```python
from build123d import *

# Parameters (mm, degrees)
SKETCH1_W           = 128.27
SKETCH1_H           = 143.764
BOSS_EXTRUDE1_DEPTH = 45.72
SKETCH3_W           = 115.57
SKETCH3_H           = 131.064
CUT_EXTRUDE1_DEPTH  = 41.91
SKETCH4_W           = 77.47
SKETCH4_H           = 26.67
CUT_EXTRUDE2_DEPTH  = 190.754
SKETCH5_W           = 113.284
SKETCH5_H           = 46.99
CUT_EXTRUDE3_DEPTH  = 190.754
SKETCH6_R           = 2.794
CUT_EXTRUDE4_DEPTH  = 199.019188454
SKETCH7_R           = 5.842
SKETCH7_R_2         = 2.794
BOSS_EXTRUDE2_DEPTH = 45.72
BOSS_EXTRUDE3_START = -45.72
SKETCH8_R           = 5.842
SKETCH8_R_2         = 2.794
BOSS_EXTRUDE3_DEPTH = 45.72
SKETCH9_R           = 5.842
SKETCH9_R_2         = 2.794
BOSS_EXTRUDE4_DEPTH = 45.72
BOSS_EXTRUDE5_START = -45.72
SKETCH10_R          = 5.842
SKETCH10_R_2        = 2.794
BOSS_EXTRUDE5_DEPTH = 45.72


with BuildPart() as part:
    # Sketch1 → Boss-Extrude1 (new body)
    with BuildSketch(Plane(origin=(0, 0, 0), x_dir=(1, 0, 0), z_dir=(0, 1, 0))):
        with Locations((64.135, 71.882)):
            Rectangle(SKETCH1_W, SKETCH1_H)
    extrude(amount=BOSS_EXTRUDE1_DEPTH)

    # Sketch3 → Cut-Extrude1 (cut)
    with BuildSketch(Plane.XZ):
        with Locations((64.135, -71.882)):
            Rectangle(SKETCH3_W, SKETCH3_H)
    extrude(amount=-CUT_EXTRUDE1_DEPTH, mode=Mode.SUBTRACT)

    # Sketch4 → Cut-Extrude2 (cut)
    with BuildSketch(Plane(origin=(0, 0, -143.764), x_dir=(-1, 0, 0), z_dir=(0, 0, -1))):
        with Locations((-64.135, 22.606)):
            Rectangle(SKETCH4_W, SKETCH4_H)
    extrude(amount=-CUT_EXTRUDE2_DEPTH, mode=Mode.SUBTRACT)

    # Sketch5 → Cut-Extrude3 (cut)
    with BuildSketch(Plane(origin=(128.27, 0, 0), x_dir=(0, 0, -1), z_dir=(1, 0, 0))):
        with Locations((71.882, 13.335)):
            Rectangle(SKETCH5_W, SKETCH5_H)
    extrude(amount=-CUT_EXTRUDE3_DEPTH, mode=Mode.SUBTRACT)

    # Sketch6 → Cut-Extrude4 (cut, through all)
    with BuildSketch(Plane(origin=(0, 0, 0), x_dir=(-1, 0, 0), z_dir=(0, -1, 0))):
        with Locations(Location((-3.81, 3.81, 0), (0, 0, 90))):
            Circle(SKETCH6_R)
        with Locations(Location((-124.46, 3.81, 0), (0, 0, 90))):
            Circle(SKETCH6_R)
        with Locations(Location((-3.81, 139.954, 0), (0, 0, 90))):
            Circle(SKETCH6_R)
        with Locations(Location((-124.46, 139.954, 0), (0, 0, 90))):
            Circle(SKETCH6_R)
    extrude(amount=-CUT_EXTRUDE4_DEPTH, mode=Mode.SUBTRACT)

    # Sketch7 → Boss-Extrude2 (add, through all)
    with BuildSketch(Plane.XZ):
        with Locations((3.81, -3.81)):
            Circle(SKETCH7_R)
        with Locations(Location((3.81, -3.81, 0), (0, 0, 270))):
            Circle(SKETCH7_R_2, mode=Mode.SUBTRACT)
    extrude(amount=-BOSS_EXTRUDE2_DEPTH)

    # Sketch8 → Boss-Extrude3 (add)
    with BuildSketch(Plane.XZ.offset(BOSS_EXTRUDE3_START)):
        with Locations((124.46, -3.81)):
            Circle(SKETCH8_R)
        with Locations(Location((124.46, -3.81, 0), (0, 0, 270))):
            Circle(SKETCH8_R_2, mode=Mode.SUBTRACT)
    extrude(amount=BOSS_EXTRUDE3_DEPTH)

    # Sketch9 → Boss-Extrude4 (add, through all)
    with BuildSketch(Plane.XZ):
        with Locations((3.81, -139.954)):
            Circle(SKETCH9_R)
        with Locations(Location((3.81, -139.954, 0), (0, 0, 270))):
            Circle(SKETCH9_R_2, mode=Mode.SUBTRACT)
    extrude(amount=-BOSS_EXTRUDE4_DEPTH)

    # Sketch10 → Boss-Extrude5 (add)
    with BuildSketch(Plane.XZ.offset(BOSS_EXTRUDE5_START)):
        with Locations((124.46, -139.954)):
            Circle(SKETCH10_R)
        with Locations(Location((124.46, -139.954, 0), (0, 0, 270))):
            Circle(SKETCH10_R_2, mode=Mode.SUBTRACT)
    extrude(amount=BOSS_EXTRUDE5_DEPTH)


solid = part.part
```
The listing builds one solid part. Answer for the finished solid, in the listing's coordinates (mm). A direction names the side the tool comes from. Give positions to 0.01 mm unless a question says otherwise; leave off trailing zeros. Order: outer loops, then holes, each group sorted by start corner. A loop starts at its lowest first (then second) coordinate and runs counter-clockwise, first axis right, second up. Notation, with made-up numbers: (27.25, 89) - (61.25, 89) arc R9 ccw to (61.25, 101) - close; hole circle Ø3 at (66.25, 48). An arc over 180 degrees is marked (long way). Use one line per item in the form item = value. Start each with the question number.
(1) Consider line 1 (X direction, y = 26, z = -3.81); line 2 (X direction, y = 5.5, z = -6); line 3 (Y direction, x = 88, z = -5). Determine where each line is inside the solid, lowest interval first. Write a range as from..to.
(2) Flat-ended cylindrical pins translate along their axes: pin 1 Ø6 at (x, z) = (37.5, -123.5) entering from -Y; pin 2 Ø4 at (y, z) = (40, -71) entering from -X; pin 3 Ø3 at (y, z) = (27, -142) entering from +X. Find the tip coordinate at first contact, or state that the pin passes through.
(3) For faces 1 (the flat face through (63, 7, -137.414)), 2 (the flat face through (102.87, 22, -3)), 3 (the flat face through (125, 36.83, -71)), determine the directions among +Z, -Z, +X, -X, +Y, -Y from which every point of the face is accessible in a straight line to the end or side of a thin tool.
(4) A cutting plane is placed at B-B, the plane x = 56.5. Write down the section's boundary in (y, z), then the cut area to 3 significant figures.
(5) A cutting plane is placed at D-D, the plane z = -115. Write down the section's boundary in (x, y), then the cut area to 3 significant figures.
(6) The mould has two halves that part along X. Classify faces 4 (the flat face through (25.4, 22, -3)), 5 (the flat face through (128.27, 38, -62)), 6 (the flat face through (63, 0, -139)): released by +X, released by -X, zero draft, split by the parting line, or undercut.
(7) A cutting plane is placed at A-A, the plane z = -3.81. Write down the section's boundary in (x, y), then the cut area to 3 significant figures.
(8) A cutting plane is placed at C-C, the plane y = 11. State how many separate pieces and enclosed holes the cut face has, then the cut area to 3 significant figures.
Ans:
q1.line_1 = -2.03..1.02, 6.6..25.4, 102.87..121.67, 127.25..130.3
q1.line_2 = -1.61..2.07, 5.55..122.72, 126.2..129.88
q1.line_3 = 0..9.27, 35.94..45.72
q2.pin_1 = 41.91
q2.pin_2 = 0
q2.pin_3 = 130.28
q3.face_1 = -Y
q3.face_2 = +Z, -Z
q3.face_3 = +X, -X, -Y
q4.outline = (0, -143.76) - (9.27, -143.76) - (9.27, -137.41) - (0, -137.41) - close; (0, -6.35) - (9.27, -6.35) - (9.27, 0) - (0, 0) - close; (35.94, -143.76) - (45.72, -143.76) - (45.72, 0) - (35.94, 0) - (35.94, -6.35) - (41.91, -6.35) - (41.91, -137.41) - (35.94, -137.41) - close
q4.area = 741 mm^2
q5.outline = (0, 36.83) - (6.35, 36.83) - (6.35, 41.91) - (121.92, 41.91) - (121.92, 36.83) - (128.27, 36.83) - (128.27, 45.72) - (0, 45.72) - close
q5.area = 553 mm^2
q6.face_4 = undercut
q6.face_5 = released by +X
q6.face_6 = zero draft
q7.outline = (-2.03, 0) - (1.02, 0) - (1.02, 45.72) - (-2.03, 45.72) - close; (6.6, 0) - (121.67, 0) - (121.67, 45.72) - (6.6, 45.72) - close; (127.25, 0) - (130.3, 0) - (130.3, 45.72) - (127.25, 45.72) - close; hole (25.4, 9.27) - (102.87, 9.27) - (102.87, 35.94) - (25.4, 35.94) - close
q7.area = 3,470 mm^2
q8.separate_pieces = 4
q8.enclosed_holes = 4
q8.area = 890 mm^2
